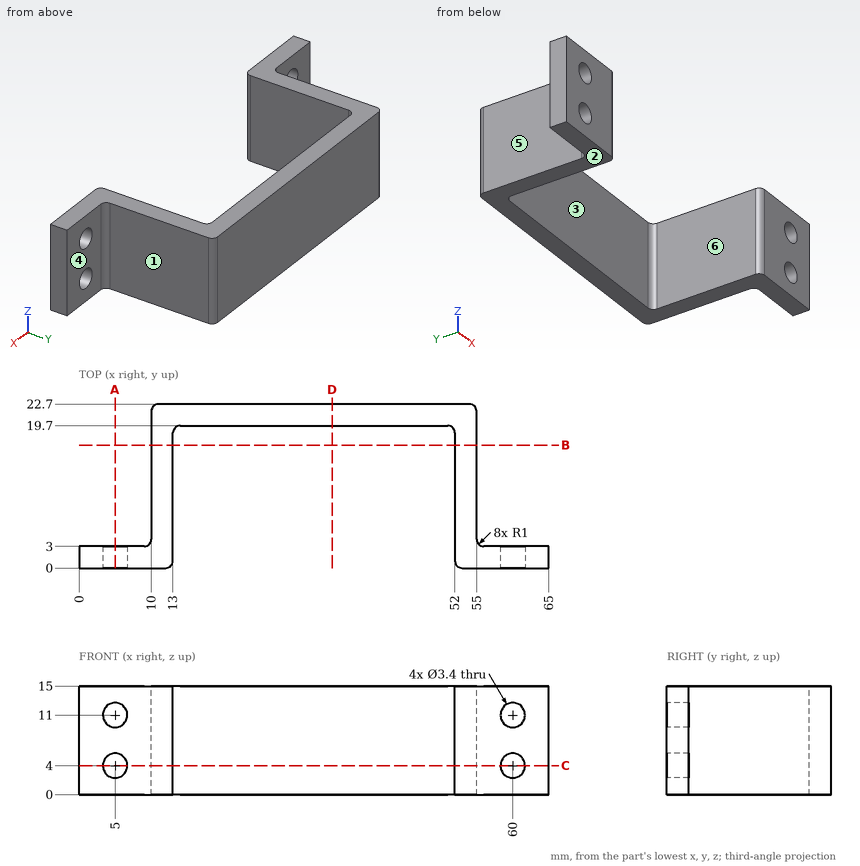
Part print with two shaded views. Sizes in mm from the minimum x, y, z corner. A direction names the side the tool comes from. Give positions to 0.01 mm unless a question says otherwise; leave off trailing zeros. Write each loop counter-clockwise with the first axis right and the second up, starting at its lowest first coordinate (ties: lowest second). Pieces come first, ordered by that corner, then holes.
1) Cut at D-D on x = 35. Write the cut outline in (y, z).
Resolved:
outline: (19.7, 0) - (22.7, 0) - (22.7, 15) - (19.7, 15) - close
2) Pin check, flat tips, straight feed: pin 1 (2 mm diameter, centred on x = 5, z = 11, fed in from -Y); pin 2 (4.5 mm diameter, centred on x = 62, z = 10, fed in from +Y); pin 3 (4.5 mm diameter, centred on y = 13, z = 11, fed in from +X); pin 4 (3 mm diameter, centred on x = 55.5, z = 13, fed in from +Y). Stop position of each tip, or through.
Resolved:
pin 1: passes through
pin 2: stops at y = 3
pin 3: stops at x = 55
pin 4: stops at y = 22.7
3) Cut at C-C on z = 4. Write the cut outline in (x, y), then the cut area to 3 significant figures.
Resolved:
outline: (0, 0) - (3.3, 0) - (3.3, 3) - (0, 3) - close; (6.7, 0) - (12, 0) arc R1 ccw to (13, 1) - (13, 18.7) arc R1 cw to (14, 19.7) - (51, 19.7) arc R1 cw to (52, 18.7) - (52, 1) arc R1 ccw to (53, 0) - (58.3, 0) - (58.3, 3) - (56, 3) arc R1 cw to (55, 4) - (55, 21.7) arc R1 ccw to (54, 22.7) - (11, 22.7) arc R1 ccw to (10, 21.7) - (10, 4) arc R1 cw to (9, 3) - (6.7, 3) - close; (61.7, 0) - (65, 0) - (65, 3) - (61.7, 3) - close
area: 293 mm2
4) Cut at B-B on y = 17. Write the cut outline in (x, z).
Resolved:
outline: (10, 0) - (13, 0) - (13, 15) - (10, 15) - close; (52, 0) - (55, 0) - (55, 15) - (52, 15) - close
5) Probe L1, parallel to Z at x = 5, y = 1.4; L2, parallel to X at y = 1.8, z = 4; L3, parallel to X at y = 17.75, z = 11.5. List the from-to ranges inside material, lowest first.
Resolved:
L1: z = 0 to 2.3, 5.7 to 9.3, 12.7 to 15
L2: x = 0 to 3.3, 6.7 to 13, 52 to 58.3, 61.7 to 65
L3: x = 10 to 13, 52 to 55
6) Which spindle directions (+Z, -Z, +X, -X, +Y, -Y) get a long thin tool onto all of the face, cutting with end or side? Do the marked faces 4, 5 and 6. Say none if no direction does.
Resolved:
face 4: +Z, -Z, +X, +Y
face 5: +Z, -Z, -X, +Y
face 6: +Z, -Z, -Y
7) Two-plate mould, pull along X, no slides. Class the marked faces 1, 2 and 3: released by +X, released by -X, zero draft, split by the parting line, or undercut.
Resolved:
face 1: released by +X
face 2: zero draft
face 3: undercut
8) Cut at A-A on x = 5. Write the cut outline in (y, z).
Resolved:
outline: (0, 0) - (3, 0) - (3, 2.3) - (0, 2.3) - close; (0, 5.7) - (3, 5.7) - (3, 9.3) - (0, 9.3) - close; (0, 12.7) - (3, 12.7) - (3, 15) - (0, 15) - close
